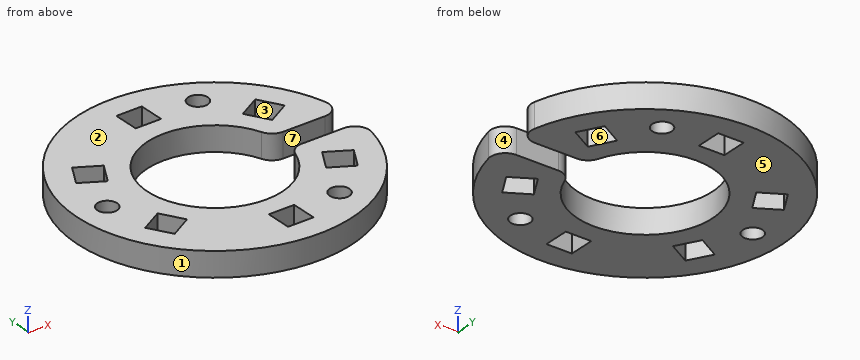
```python
from build123d import *

# Parameters (mm, degrees)
SKETCH1_R           = 2
SKETCH1_W           = 5.2
SKETCH1_H           = 5.2
BOSS_EXTRUDE1_DEPTH = 5
CONG_2_R            = 3


with BuildPart() as part:
    # Sketch1 → Boss-Extrude1 (new body)
    with BuildSketch(Plane.XY):
        with BuildLine():
            Line((27.888169535, 2.5), (13.520817283, 2.5))
            ThreePointArc((13.520817283, 2.5), (-13.75, 0), (13.520817283, -2.5))
            Line((13.520817283, -2.5), (27.888169535, -2.5))
            ThreePointArc((27.888169535, -2.5), (-28, 0), (27.888169535, 2.5))
        make_face()
        with Locations((11, 19.052558883)):
            Circle(SKETCH1_R, mode=Mode.SUBTRACT)
        with Locations((11, -19.052558883)):
            Circle(SKETCH1_R, mode=Mode.SUBTRACT)
        with Locations((-22, 0)):
            Circle(SKETCH1_R, mode=Mode.SUBTRACT)
        with Locations((0, 20.5)):
            Rectangle(SKETCH1_W, SKETCH1_H, mode=Mode.SUBTRACT)
        Polygon((21.305186827, 9.29833395), (16.801854728, 6.69833395), (14.201854728, 11.20166605), (18.705186827, 13.80166605), align=None, mode=Mode.SUBTRACT)
        Polygon((18.705186827, -13.80166605), (14.201854728, -11.20166605), (16.801854728, -6.69833395), (21.305186827, -9.29833395), align=None, mode=Mode.SUBTRACT)
        with Locations((0, -20.5)):
            Rectangle(SKETCH1_W, SKETCH1_H, mode=Mode.SUBTRACT)
        Polygon((-21.305186827, -9.29833395), (-16.801854728, -6.69833395), (-14.201854728, -11.20166605), (-18.705186827, -13.80166605), align=None, mode=Mode.SUBTRACT)
        Polygon((-18.705186827, 13.80166605), (-14.201854728, 11.20166605), (-16.801854728, 6.69833395), (-21.305186827, 9.29833395), align=None, mode=Mode.SUBTRACT)
    extrude(amount=BOSS_EXTRUDE1_DEPTH)

    # Congé2
    cong_2_edges = [part.edges().sort_by_distance(p)[0] for p in [
        (27.888169535, 2.5, 2.5),
        (13.520817283, 2.5, 2.5),
        (13.520817283, -2.5, 2.5),
        (27.888169535, -2.5, 2.5),
    ]]
    fillet(cong_2_edges, radius=CONG_2_R)


solid = part.part
```
Verification items for the finished model (mm, model axes). Face numbers are marked on the shaded views. A direction names the side the tool comes from. Coordinates: 2 decimals unless noted, no trailing zeros. Loops run counter-clockwise (first coordinate to the right, second up) from the corner with the lowest first, then second, coordinate; pieces in that order, holes last. Notation, with made-up numbers: (53.25, -1.5) - (75.25, -1.5) arc R15 cw to (75.25, 18.5) - close; hole circle Ø10 at (-2, 47). An arc over 180 degrees is marked (long way). Return JSON: item names as keys, results as strings.
1. Section check B-B, the plane y = 0. Record the boundary of the cut face in (x, z), then the cut area to 4 significant figures.
Established:
{"outline": "(-28, 0) - (-24, 0) - (-24, 5) - (-28, 5) - close; (-20, 0) - (-13.75, 0) - (-13.75, 5) - (-20, 5) - close", "area": "51.25 mm2"}
2. Go/stop test with flat-tipped pins: pin 1 (1.5 mm diameter, centred on x = 1, z = 2, fed in from +Y); pin 2 (1.5 mm diameter, centred on y = 21, z = 1.5, fed in from +X); pin 3 (2 mm diameter, centred on y = -4, z = 2, fed in from +X). Record where each tip stops, or that it passes through.
Established:
{"pin 1": "stops at y = 28", "pin 2": "stops at x = 19.34", "pin 3": "stops at x = 27.35"}
3. Thickness scan on L1, parallel to Y at x = 0, z = 3.6; L2, parallel to Y at x = 11, z = 2.8; L3, parallel to X at y = 18.5, z = 3.55. Record the ranges inside material, lowest first.
Established:
{"L1": "y = -28 to -23.1, -17.9 to -13.75, 13.75 to 17.9, 23.1 to 28", "L2": "y = -25.75 to -21.05, -17.05 to -8.25, 8.25 to 17.05, 21.05 to 25.75", "L3": "x = -21.02 to -2.6, 2.6 to 9.08, 12.92 to 21.02"}
4. Section check A-A, the plane x = 0. Record the boundary of the cut face in (y, z).
Established:
{"outline": "(-28, 0) - (-23.1, 0) - (-23.1, 5) - (-28, 5) - close; (-17.9, 0) - (-13.75, 0) - (-13.75, 5) - (-17.9, 5) - close; (13.75, 0) - (17.9, 0) - (17.9, 5) - (13.75, 5) - close; (23.1, 0) - (28, 0) - (28, 5) - (23.1, 5) - close"}
5. Mould release check, pull along Y, two halves, no side actions. Record for the marked faces 1, 2, 3 and 4: +Y half, -Y half, draft (parallel to the pull), parting line (faces both ways), or undercut.
Established:
{"face 1": "parting line", "face 2": "draft", "face 3": "undercut", "face 4": "undercut"}
6. Section check C-C, the plane y = -8. Record the boundary of the cut face in (x, z), then the cut area to 3 significant figures.
Established:
{"outline": "(-26.83, 0) - (-19.06, 0) - (-19.06, 5) - (-26.83, 5) - close; (-16.05, 0) - (-11.18, 0) - (-11.18, 5) - (-16.05, 5) - close; (11.18, 0) - (16.05, 0) - (16.05, 5) - (11.18, 5) - close; (19.06, 0) - (26.83, 0) - (26.83, 5) - (19.06, 5) - close", "area": "126 mm2"}
7. Tool access check on the marked faces 5, 6 and 7. Record the directions out of +Z, -Z, +X, -X, +Y, -Y that give a thin tool (end or side, any length) a straight path to the whole face; none if there is none.
Established:
{"face 5": "-Z, +X, -X, +Y, -Y", "face 6": "+Z, -Z", "face 7": "+Z, -Z, +X"}
8. Section check D-D, the plane x = -6.5. Record the boundary of the cut face in (y, z), then the cut area to 3 significant figures.
Established:
{"outline": "(-27.24, 0) - (-12.12, 0) - (-12.12, 5) - (-27.24, 5) - close; (12.12, 0) - (27.24, 0) - (27.24, 5) - (12.12, 5) - close", "area": "151 mm2"}
